Verification items for this drawing (mm, ordinates from the low corner). A direction names the side the tool comes from. Give positions to 0.01 mm unless a question says otherwise; leave off trailing zeros. Write each loop counter-clockwise with the first axis right and the second up, starting at its lowest first coordinate (ties: lowest second). Pieces come first, ordered by that corner, then holes. Notation, with made-up numbers: M 6,80.5 L 19,80.5 A29 ccw 19,100.5 Z; hole C -7.5,36 d8. An arc over 180 degrees is marked long. Write each question's results on one line, items separated by ' | '.
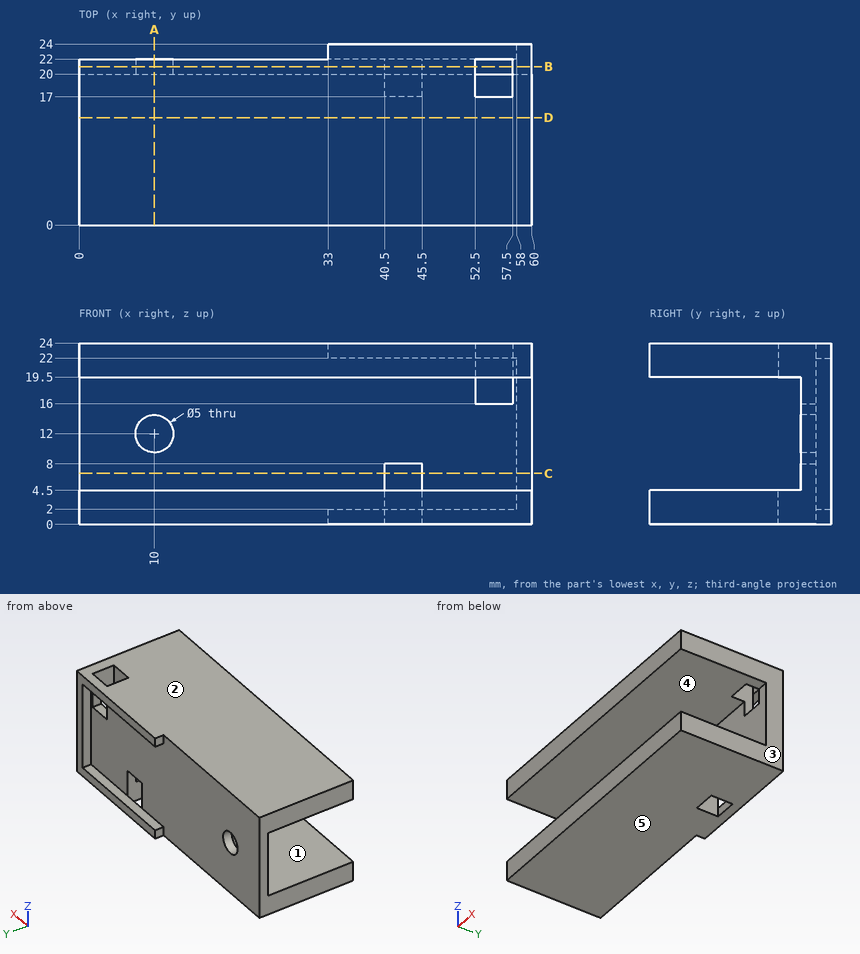
Q1. Access from +Z, -Z, +X, -X, +Y, -Y to the whole of each face (thin tool, end or side, straight path). Record for the marked faces 1 and 2.
Answer key:
face 1: +X, -X, -Y | face 2: +Z, +X, -X, +Y, -Y
Q2. Section check C-C (z = 6.75). Enter the section's corners in (x, y).
Answer key:
outline: M 0,20 L 40.5,20 L 40.5,22 L 0,22 Z; M 45.5,20 L 60,20 L 60,24 L 58,24 L 58,22 L 45.5,22 Z
Q3. Section check B-B (y = 21). Enter the section's corners in (x, z).
Answer key:
outline: M 0,0 L 40.5,0 L 40.5,8 L 45.5,8 L 45.5,0 L 60,0 L 60,24 L 57.5,24 L 57.5,16 L 52.5,16 L 52.5,24 L 0,24 Z; hole C 10,12 d5
Q4. Release check for a two-part mould opening along Z. For the marked faces 3, 4 and 5 record: released by +Z, released by -Z, zero draft, split by the parting line, or undercut.
Answer key:
face 3: zero draft | face 4: undercut | face 5: released by -Z
Q5. Depth check by flat-ended pin: P1, Ø1, axis at x = 55.5, y = 20.5, coming from the +Z side; P2, Ø1, axis at y = 23, z = 23, coming from the -X side; P3, Ø1, axis at x = 20.5, z = 21, coming from the +Y side. Enter the tip coordinate at first touch or a pass-through.
Answer key:
P1: stops at z = 16 | P2: stops at x = 33 | P3: stops at y = 22
Q6. Section check A-A (x = 10). Enter the section's corners in (y, z), then the cut area to 3 significant figures.
Answer key:
outline: M 0,0 L 22,0 L 22,9.5 L 20,9.5 L 20,4.5 L 0,4.5 Z; M 0,19.5 L 20,19.5 L 20,14.5 L 22,14.5 L 22,24 L 0,24 Z | area: 218 mm2
Q7. Material ranges on probe 1 along Z at (x, y) = (10, 20.55); probe 2 along X at (y, z) = (20.9, 12); probe 3 along Z at (x, y) = (28, 19), recorded low to high. Write a range as [from, to].
Answer key:
probe 1: z = [0, 9.5], [14.5, 24] | probe 2: x = [0, 7.5], [12.5, 60] | probe 3: z = [0, 4.5], [19.5, 24]
Q8. Section check D-D (y = 14.25). Enter the section's corners in (x, z), then the cut area to 3 significant figures.
Answer key:
outline: M 0,0 L 60,0 L 60,4.5 L 0,4.5 Z; M 0,19.5 L 60,19.5 L 60,24 L 0,24 Z | area: 540 mm2
